Study the drawing (mm; zero at the part's minimum x, y, z) and answer. Round coordinates to 2 decimals unless told otherwise and drop trailing zeros. Write each loop counter-clockwise with the first axis right and the second up, starting at its lowest first coordinate (ties: lowest second). Pieces come first, ordered by that corner, then holes. Notation, with made-up numbers: (89, 58) -> (93, 58) arc R26 ccw to (93, 93) -> close; hole circle Ø8 at (67, 49). An arc over 180 degrees is marked (long way). Return JSON: item names as keys, results as strings.
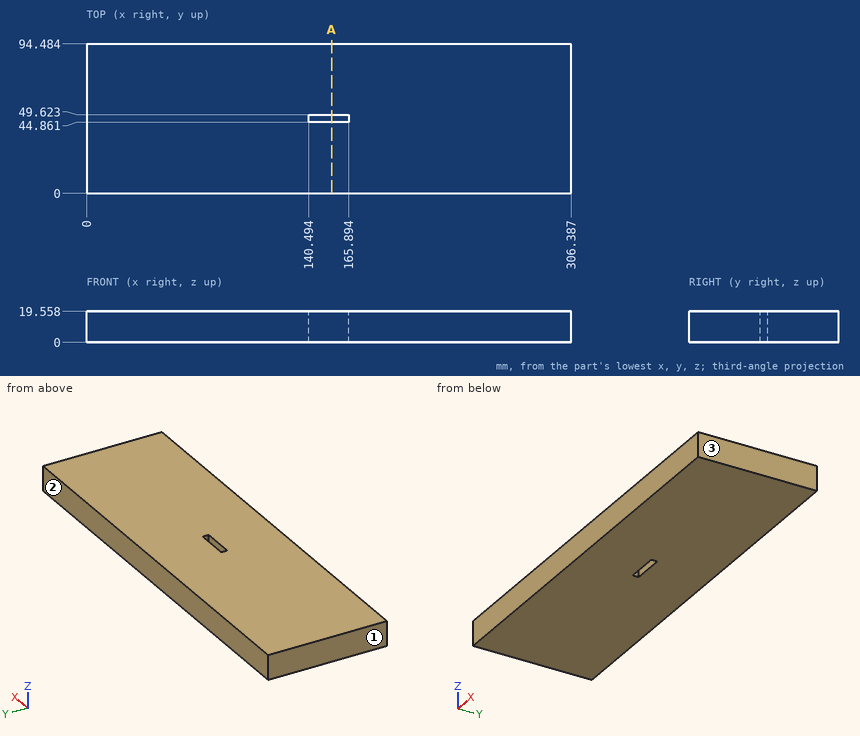
Item 1: Section A-A (x = 155) is taken. Give the vertices of the cut face in (y, z), then the cut area to 4 significant figures.
Worked answers:
{"outline": "(0, 0) -> (44.86, 0) -> (44.86, 19.56) -> (0, 19.56) -> close; (49.62, 0) -> (94.48, 0) -> (94.48, 19.56) -> (49.62, 19.56) -> close", "area": "1,755 mm2"}
Item 2: A straight line is drawn through the part: L1, parallel to Y at x = 156.5, z = 17. Find the intervals that lie inside material, in ascending order. Write a range as [from, to].
Worked answers:
{"L1": "y = [0, 44.86], [49.62, 94.48]"}
Item 3: For a pull along X with two mould halves and no side action, classify the marked faces 1, 2 and 3 as released by +X, released by -X, zero draft, split by the parting line, or undercut.
Worked answers:
{"face 1": "released by -X", "face 2": "zero draft", "face 3": "released by +X"}
